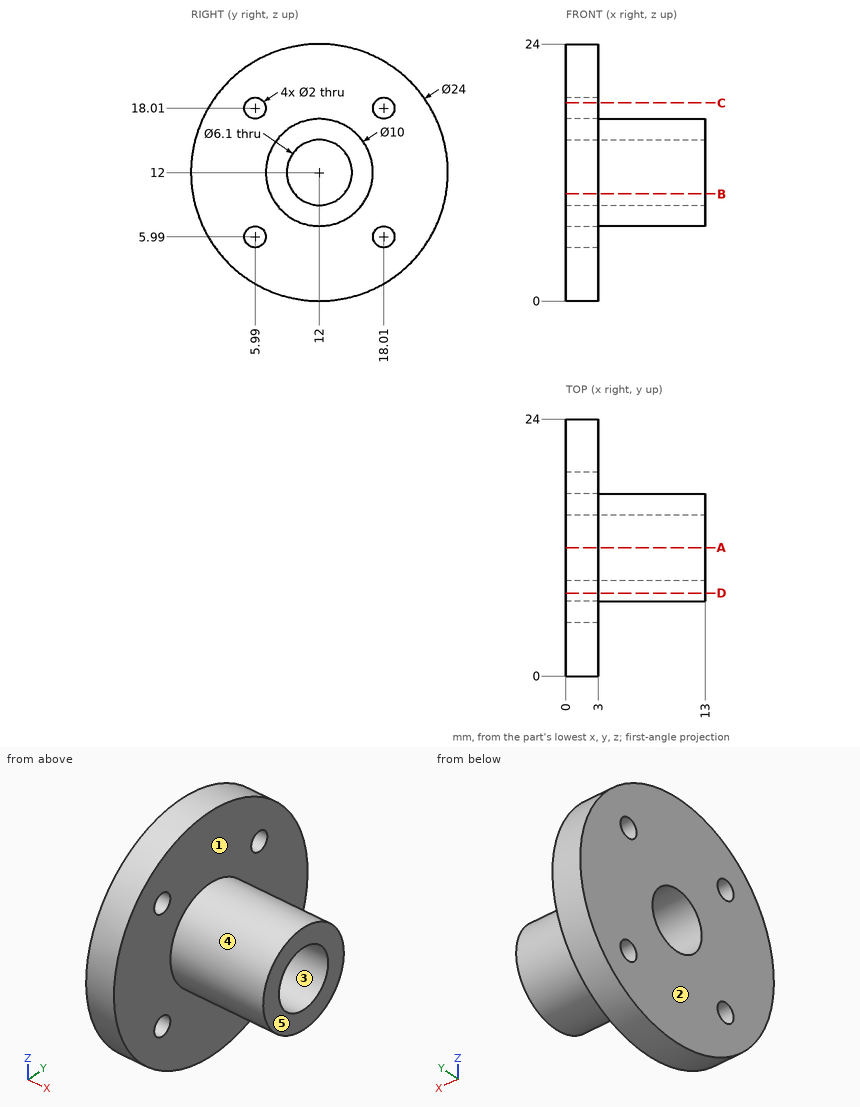
Study the drawing (mm; zero at the part's minimum x, y, z) and answer. A direction names the side the tool comes from. Round coordinates to 2 decimals unless told otherwise and drop trailing zeros. Loops run counter-clockwise (first coordinate to the right, second up) from the corner with the lowest first, then second, coordinate; pieces in that order, holes last.
Q1. Section C-C, the plane z = 18.5 is taken. Determine the outline of the cut face in (x, y).
Q2. Section D-D, the plane y = 7.75 is taken. Determine the outline of the cut face in (x, z), then the cut area to 3 significant figures.
Q3. Which of the six approach directions +Z, -Z, +X, -X, +Y, -Y give full straight-line access (tool end or side, diameter ignored) to the marked faces 1 and 2?
Q4. Find the intervals of material crossed by line 1 (Y direction, x = 7, z = 12); line 2 (X direction, y = 8, z = 22.75); line 3 (Z direction, x = 1.5, y = 14), in increasing order.
Q5. Section B-B, the plane z = 10 is taken. Determine the outline of the cut face in (x, y), then the cut area to 3 significant figures.
Q6. For a pull along Z with two mould halves and no side action, classify the marked faces 3, 4 and 5 as released by +Z, released by -Z, zero draft, split by the parting line, or undercut.
Q7. Given pin 1 Ø1 at (y, z) = (13.5, 13.5) entering from +X; pin 2 Ø6 at (x, y) = (11, 18.5) entering from +Z; pin 3 Ø3 at (y, z) = (18.01, 18.01) entering from +X; pin 4 Ø2 at (x, y) = (3, 19) entering from -Z, each flat-ended and moving along its own axis, determine where each tip first touches the part or whether it passes through.
Q8. Section A-A, the plane y = 12 is taken. Determine the outline of the cut face in (x, z).
Completed:
1. outline: (0, 1.91) - (3, 1.91) - (3, 5.12) - (0, 5.12) - close; (0, 6.86) - (3, 6.86) - (3, 17.14) - (0, 17.14) - close; (0, 18.88) - (3, 18.88) - (3, 22.09) - (0, 22.09) - close
2. outline: (0, 0.78) - (3, 0.78) - (3, 9.37) - (13, 9.37) - (13, 14.63) - (3, 14.63) - (3, 23.22) - (0, 23.22) - close
2. area: 120 mm2
3. face 1: +X
3. face 2: +Z, -Z, -X, +Y, -Y
4. line 1: y = 7 to 8.95, 15.05 to 17
4. line 2: x = 0 to 3
4. line 3: z = 0.17 to 9.7, 14.3 to 23.83
5. outline: (0, 0.17) - (3, 0.17) - (3, 7.42) - (13, 7.42) - (13, 9.7) - (0, 9.7) - close; (0, 14.3) - (13, 14.3) - (13, 16.58) - (3, 16.58) - (3, 23.83) - (0, 23.83) - close
5. area: 103 mm2
6. face 3: undercut
6. face 4: split by the parting line
6. face 5: zero draft
7. pin 1: passes through
7. pin 2: stops at z = 15.57
7. pin 3: stops at x = 3
7. pin 4: stops at z = 1.61
8. outline: (0, 0) - (3, 0) - (3, 7) - (13, 7) - (13, 8.95) - (0, 8.95) - close; (0, 15.05) - (13, 15.05) - (13, 17) - (3, 17) - (3, 24) - (0, 24) - close
